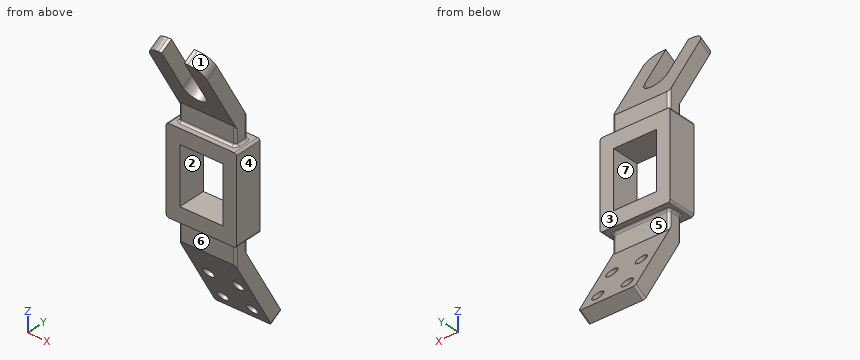
```python
from build123d import *

# Parameters (mm, degrees)
SKETCH_1_W          = 62
SKETCH_1_H          = 76
SKETCH_1_W_2        = 38
SKETCH_1_H_2        = 50
EXTRUDE_1_DEPTH     = 12.5
EXTRUDE_2_DEPTH     = 25
SKETCH_3_R          = 5
CUT_EXTRUDE_3_DEPTH = 151.634898624
CUT_EXTRUDE_4_DEPTH = 161.843921561
FILLET_1_R          = 12
FILLET_2_R          = 2
FILLET_3_R          = 2


with BuildPart() as part:
    # 草圖1 → 伸長1 (new, symmetric)
    with BuildSketch(Plane(origin=(0, 0, 0), x_dir=(1, 0, 0), z_dir=(0, 1, 0))):
        Rectangle(SKETCH_1_W, SKETCH_1_H)
        Rectangle(SKETCH_1_W_2, SKETCH_1_H_2, mode=Mode.SUBTRACT)
    extrude(amount=EXTRUDE_1_DEPTH, both=True)

    # 草圖2 → 伸長2 (add, symmetric)
    with BuildSketch(Plane(origin=(0, 0, 0), x_dir=(0, 0, -1), z_dir=(1, 0, 0))):
        Polygon((38, 6), (54.784609691, 6), (117.817930688, 42.392304845), (123.817930688, 32), (58, -6), (38, -6), align=None)
        Polygon((-38, 6), (-57, 6), (-122.817930688, -32), (-116.817930688, -42.392304845), (-53.784609691, -6), (-38, -6), align=None)
    extrude(amount=EXTRUDE_2_DEPTH, both=True)

    # 草圖3 → 伸長3 (cut, through all)
    with BuildSketch(Plane(origin=(0, -19.222431864, -11.098076211), x_dir=(1, 0, 0), z_dir=(0, 0.8660254037844377, 0.5000000000000018))):
        with Locations(Location((-13, 111.229473419, 0), (0, 0, 270))):
            Circle(SKETCH_3_R)
        with Locations(Location((13, 111.229473419, 0), (0, 0, 270))):
            Circle(SKETCH_3_R)
        with Locations(Location((-13, 81.229473419, 0), (0, 0, 270))):
            Circle(SKETCH_3_R)
        with Locations(Location((13, 81.229473419, 0), (0, 0, 270))):
            Circle(SKETCH_3_R)
    extrude(amount=-CUT_EXTRUDE_3_DEPTH, mode=Mode.SUBTRACT)

    # 草圖4 → 伸長4 (cut, through all)
    with BuildSketch(Plane(origin=(0, 29.181724008, 16.848076211), x_dir=(1, 0, 0), z_dir=(0, 0.8660254037844377, 0.5000000000000014))):
        with BuildLine():
            Line((-10, -122.363448016), (-10, -77.363448016))
            ThreePointArc((-10, -77.363448016), (0, -67.363448016), (10, -77.363448016))
            Line((10, -77.363448016), (10, -122.363448016))
            Line((10, -122.363448016), (-10, -122.363448016))
        make_face()
    extrude(amount=-CUT_EXTRUDE_4_DEPTH, mode=Mode.SUBTRACT)

    # 圓角1
    fillet_1_edges = [part.edges().sort_by_distance(p)[0] for p in [
        (-25, -37.196152423, 119.817930688),
        (25, -37.196152423, 119.817930688),
    ]]
    fillet(fillet_1_edges, radius=FILLET_1_R)

    # 圓角2
    fillet_2_edges = [part.edges().sort_by_distance(p)[0] for p in [
        (-25, -6, -48),
        (-25, 37.196152423, -120.817930688),
        (-25, 6, -46.392304845),
        (25, -6, -48),
        (25, 37.196152423, -120.817930688),
        (25, 6, -46.392304845),
        (-25, 6, 47.5),
        (-25, -6, 45.892304845),
        (25, 6, 47.5),
        (25, -6, 45.892304845),
        (-31, 0, -38),
        (31, 0, -38),
        (31, 0, 38),
        (-31, 0, 38),
    ]]
    fillet(fillet_2_edges, radius=FILLET_2_R)

    # 圓角3
    fillet_3_edges = [part.edges().sort_by_distance(p)[0] for p in [
        (0, -6, -38),
        (-25, 0, -38),
        (0, 6, -38),
        (25, 0, -38),
        (0, -6, 38),
        (-25, 0, 38),
        (0, 6, 38),
        (25, 0, 38),
        (-24.414213562, -5.414213562, -38),
        (-24.414213562, 5.414213562, -38),
        (24.414213562, -5.414213562, -38),
        (24.414213562, 5.414213562, -38),
        (-24.414213562, -5.414213562, 38),
        (-24.414213562, 5.414213562, 38),
        (24.414213562, -5.414213562, 38),
        (24.414213562, 5.414213562, 38),
    ]]
    fillet(fillet_3_edges, radius=FILLET_3_R)


solid = part.part
```
Read the model definition and answer for the solid it produces. Units are mm, in the model's axes. Face numbers are marked on the shaded views. A direction names the side the tool comes from. Round coordinates to 2 decimals unless told otherwise and drop trailing zeros. Write each loop counter-clockwise with the first axis right and the second up, starting at its lowest first coordinate (ties: lowest second). Pieces come first, ordered by that corner, then holes. Notation, with made-up numbers: (-14, 67) -> (20, 67) arc R28 cw to (20, 104) -> close; hole circle Ø4 at (-39.5, 32.5). An arc over 180 degrees is marked (long way). Answer in a Markdown table with one row per item. Add a question column.
1) Determine the mould class of the marked faces 1, 2 and 3 for opening direction X: pulls with the +X half, pulls with the -X half, needs draft (parallel to the pull), parting line crosses it, or undercut.
2) Which of the six approach directions +Z, -Z, +X, -X, +Y, -Y give full straight-line access (tool end or side, diameter ignored) to the marked faces 4, 5, 6 and 7?
3) Given P1, Ø1.5, axis at x = -22.5, y = -20.5, coming from the -Z side; P2, Ø7.5, axis at x = -13, y = 5, coming from the -Z side; P3, Ø12, axis at y = -24.5, z = 78.5, coming from the +X side, each flat-ended and moving along its own axis, determine where each tip first touches the part or whether it passes through.
4) Find section D-D, the plane z = 65. Determine the outline of the cut face in (x, y), and give its area (3 significant figures).
5) Find section A-A, the plane z = 14.5. Determine the outline of the cut face in (x, y), and give its area (3 significant figures).
6) Find section C-C, the plane y = 16. State how many separate pieces and enclosed holes the cut face has, and give its area (3 significant figures).
7) Find section B-B, the plane x = -0.5. Determine the outline of the cut face in (y, z), and give its area (3 significant figures).
8) Consider line 1 (Z direction, x = -5, y = -10); line 2 (Z direction, x = 4.5, y = 7); line 3 (Y direction, x = -3.5, z = -40). Determine where each line is inside the solid, lowest interval first.
Findings below:
| question | item | result |
|---|---|---|
| 1 | face 1 | pulls with the +X half |
| 1 | face 2 | undercut |
| 1 | face 3 | needs draft |
| 2 | face 4 | +Z, -Z, +X, +Y, -Y |
| 2 | face 5 | +X, -X, +Y |
| 2 | face 6 | -Z, +X, -X, -Y |
| 2 | face 7 | +Y, -Y |
| 3 | P1 | z = 77.6 |
| 3 | P2 | z = -83.23 |
| 3 | P3 | x = 25 |
| 4 | outline | (-25, -12.48) -> (25, -12.48) -> (25, 1.38) -> (-25, 1.38) -> close |
| 4 | area | 693 mm² |
| 5 | outline | (-31, -12.5) -> (-19, -12.5) -> (-19, 12.5) -> (-31, 12.5) -> close; (19, -12.5) -> (31, -12.5) -> (31, 12.5) -> (19, 12.5) -> close |
| 5 | area | 600 mm² |
| 6 | separate pieces | 1 |
| 6 | enclosed holes | 2 |
| 6 | area | 1,020 mm² |
| 7 | outline | (-14.9, 69.2) -> (-6, 53.78) -> (-6, 40) arc R2 cw to (-8, 38) -> (-12.5, 38) -> (-12.5, 25) -> (12.5, 25) -> (12.5, 38) -> (8, 38) arc R2 cw to (6, 40) -> (6, 57) -> (-4.51, 75.2) -> close; (-12.5, -38) -> (-8, -38) arc R2 cw to (-6, -40) -> (-6, -58) -> (32, -123.82) -> (42.39, -117.82) -> (6, -54.78) -> (6, -40) arc R2 cw to (8, -38) -> (12.5, -38) -> (12.5, -25) -> (-12.5, -25) -> close |
| 7 | area | 2,210 mm² |
| 8 | line 1 | -38 to -25, 25 to 38, 60.71 to 73.56 |
| 8 | line 2 | -80.52 to -56.52, -38.27 to -25, 25 to 38.27 |
| 8 | line 3 | -6 to 6 |
